from build123d import *

# Parameters (mm, degrees)
FILLET1_R = 0.5


with BuildPart() as part:
    # Sketch1 → Revolve1 (revolve)
    with BuildSketch(Plane.XY, mode=Mode.PRIVATE) as revolve1_sk:
        with BuildLine():
            Line((0, 6.25), (0, 3.95))
            Line((0, 3.95), (51.764799444, 3.95))
            ThreePointArc((51.764799444, 3.95), (54.897363756, 4.887450418), (57, 7.391585654))
            Line((57, 7.391585654), (57, 7.8))
            ThreePointArc((57, 7.8), (54.879732128, 6.648358339), (52.5, 6.25))
            Line((52.5, 6.25), (0, 6.25))
        make_face()
    revolve(revolve1_sk.sketch.rotate(Axis((0, 0, 0), (1, 0, 0)), 90), axis=Axis((0, 0, 0), (1, 0, 0)))

    # Fillet1
    fillet1_edges = [part.edges().sort_by_distance(p)[0] for p in [
        (0, 0, -3.95),
        (0, 0, -6.25),
    ]]
    fillet(fillet1_edges, radius=FILLET1_R)


solid = part.part
CAD build for the part. Positions are in the model's coordinates, mm. Coordinates: 2 decimals unless noted, no trailing zeros. Order: outer loops, then holes, each group sorted by start corner. A loop starts at its lowest first (then second) coordinate and runs counter-clockwise, first axis right, second up.
Item 1: Band-saw the part on C-C on x = 22.5. List the corners of the cut face in (y, z).
Check sheet entries:
outline: circle Ø12.5 at (0, 0); hole circle Ø7.9 at (0, 0)
Item 2: Band-saw the part on A-A on z = 0. List the corners of the cut face in (x, y).
Check sheet entries:
outline: (0, -5.75) arc R0.5 ccw to (0.5, -6.25) - (52.5, -6.25) arc R7.31 cw to (57, -7.8) - (57, -7.39) arc R5.7 ccw to (51.76, -3.95) - (0.5, -3.95) arc R0.5 ccw to (0, -4.45) - close; (0, 4.45) arc R0.5 ccw to (0.5, 3.95) - (51.76, 3.95) arc R5.7 ccw to (57, 7.39) - (57, 7.8) arc R7.31 cw to (52.5, 6.25) - (0.5, 6.25) arc R0.5 ccw to (0, 5.75) - close
Item 3: Drill centre lines: L1, parallel to Y at x = 22, z = 0; L2, parallel to Y at x = 31.5, z = -1.25; L3, parallel to X at y = -1.25, z = 4.75. Where is each one in solid material? Low to high.
Check sheet entries:
L1: y = -6.25 to -3.95, 3.95 to 6.25
L2: y = -6.12 to -3.75, 3.75 to 6.12
L3: x = 0 to 54.93
Item 4: Pin check, flat tips, straight feed: pin 1 Ø2 at (x, z) = (35.5, -5.5) entering from -Y; pin 2 Ø2 at (y, z) = (2, 3.5) entering from +X; pin 3 Ø3 at (x, y) = (13.5, -1) entering from +Z; pin 4 Ø6 at (y, z) = (4, 3) entering from -X. Stop position of each tip, or through.
Check sheet entries:
pin 1: stops at y = -4.34
pin 2: stops at x = 55.11
pin 3: stops at z = 6.25
pin 4: stops at x = 0
Item 5: Two-plate mould, pull along Z, no slides. Class faces 1 (the face through (26.14, -1.88, 5.96)), 2 (the face through (0, 4, 3)), 3 (the face through (26.49, -2.67, -2.91)): +Z half, -Z half, draft (parallel to the pull), parting line (faces both ways), or undercut.
Check sheet entries:
face 1: parting line
face 2: draft
face 3: undercut
